from build123d import *

# Parameters (mm, degrees)
F1_DEPTH       = 30
F3_D           = 13.2
F3_CBORE_D     = 19.25
F3_CBORE_DEPTH = 12
F4_R           = 10
F5_W           = 10
F5_H           = 45
F6_DEPTH       = 30.001
F7_R           = 4.99999


# Not quite as in the source:
# - a fillet or chamfer is up to 0.001 mm smaller than in the source, because OpenCascade refuses the exact size


with BuildPart() as f1:
    # F0 (on Front) → F1 (new body)
    with BuildSketch(Plane.XZ):
        Polygon((0, 100), (0, 0), (50, 0), (50, 40), (80, 70), (110, 70), (110, 100), align=None)
    extrude(amount=-F1_DEPTH)

    # F3 (through all)
    with Locations(Plane.XZ):
        with Locations((95, 85)):
            CounterBoreHole(F3_D / 2, F3_CBORE_D / 2, F3_CBORE_DEPTH)

    # F4
    f4_edges = [f1.edges().sort_by_distance(p)[0] for p in [
        (0, 15, 100),
        (50, 15, 0),
        (110, 15, 70),
        (110, 15, 100),
        (0, 15, 0),
    ]]
    fillet(f4_edges, radius=F4_R)

    # F5 (on face) → F6 (cut, through all)
    with BuildSketch(Plane.XZ):
        with Locations((25, 50)):
            Rectangle(F5_W, F5_H)
    extrude(amount=-F6_DEPTH, mode=Mode.SUBTRACT)

    # F7 (radius 5 in the source; OpenCascade refuses exactly that, so slightly less here)
    f7_edges = [f1.edges().sort_by_distance(p)[0] for p in [
        (20, 15, 72.5),
        (30, 15, 72.5),
        (30, 15, 27.5),
        (20, 15, 27.5),
    ]]
    fillet(f7_edges, radius=F7_R)


solid = f1.part
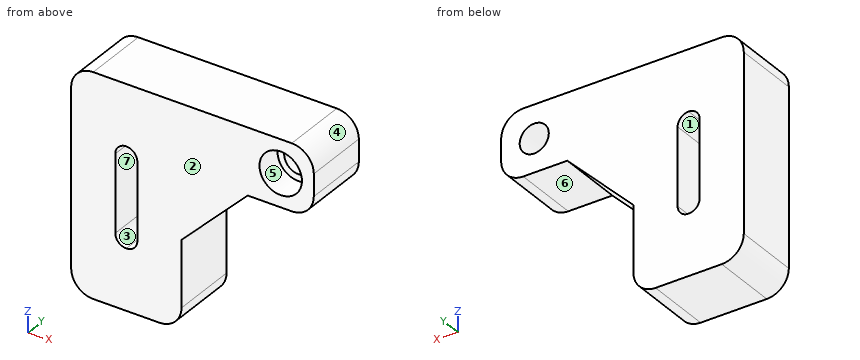
Geometry check sheet. Reference: the model listing, model coordinates, mm. Face numbers are marked on the shaded views. A direction names the side the tool comes from. Give positions to 0.01 mm unless a question says otherwise; leave off trailing zeros. Loops run counter-clockwise (first coordinate to the right, second up) from the corner with the lowest first, then second, coordinate; pieces in that order, holes last. Notation, with made-up numbers: (5, -35.75) -> (32, -35.75) arc R18 ccw to (32, -6.75) -> close; hole circle Ø7 at (27.5, 82.25). An arc over 180 degrees is marked (long way). Answer in a Markdown table with one row per item. Add a question column.
1) Cross-section at C-C on x = 95. Record the boundary of the cut face in (y, z) (3 decimals), and give its area (3 significant figures).
2) Material ranges on probe 1 along X at (y, z) = (2.75, 84.5); probe 2 along Z at (x, y) = (95, 19); probe 3 along X at (y, z) = (16.5, 36.5), recorded low to high. Write a range as from..to.
3) Cross-section at A-A on z = 85. Record the boundary of the cut face in (x, y) (3 decimals).
4) Cross-section at D-D on z = 61. Record the boundary of the cut face in (x, y), and give its area (3 significant figures).
5) Gauge pin test, flat ends, axial feed: P1, Ø16, axis at x = 86.5, y = 19.5, coming from the -Z side; P2, Ø3, axis at y = 11, z = 20, coming from the +X side; P3, Ø8, axis at x = 70, y = 4.5, coming from the -Z side. Record the tip position at first contact, or that the pin passes through.
6) Set-up check for the marked faces 5, 6 and 7: record each of +Z, -Z, +X, -X, +Y, -Y from which the full face is reachable in a straight line by a thin tool's end or side.
7) Cross-section at B-B on y = 25.5. State how many separate pieces and enclosed holes the cut face has, and give its area (3 significant figures).
8) Draft check along Z on the marked faces 1, 2, 3 and 4. Enter one of: pulls with the +Z half, pulls with the -Z half, needs draft (parallel to the pull), parting line crosses it, or undercut.
Outcome:
| question | item | result |
|---|---|---|
| 1 | outline | (0, 70) -> (30, 70) -> (30, 78.4) -> (12, 78.4) -> (12, 75.375) -> (0, 75.375) -> close; (0, 94.625) -> (12, 94.625) -> (12, 91.6) -> (30, 91.6) -> (30, 100) -> (0, 100) -> close |
| 1 | area | 431 mm^2 |
| 2 | probe 1 | x = 0..85.39, 104.61..110 |
| 2 | probe 2 | z = 70..78.4, 91.6..100 |
| 2 | probe 3 | x = 0..20, 30..50 |
| 3 | outline | (0, 0) -> (85.375, 0) -> (85.375, 12) -> (88.4, 12) -> (88.4, 30) -> (0, 30) -> close; (101.6, 12) -> (104.625, 12) -> (104.625, 0) -> (110, 0) -> (110, 30) -> (101.6, 30) -> close |
| 4 | outline | (0, 0) -> (20, 0) -> (20, 30) -> (0, 30) -> close; (30, 0) -> (71, 0) -> (71, 30) -> (30, 30) -> close |
| 4 | area | 1,830 mm^2 |
| 5 | P1 | stops at z = 68.5 |
| 5 | P2 | stops at x = 50 |
| 5 | P3 | stops at z = 56 |
| 6 | face 5 | -Y |
| 6 | face 6 | -Z, +X, +Y, -Y |
| 6 | face 7 | +Y, -Y |
| 7 | separate pieces | 1 |
| 7 | enclosed holes | 2 |
| 7 | area | 6,580 mm^2 |
| 8 | face 1 | undercut |
| 8 | face 2 | needs draft |
| 8 | face 3 | undercut |
| 8 | face 4 | pulls with the +Z half |
